from build123d import *

# Parameters (mm, degrees)
SKETCH1_W                = 37
SKETCH1_H                = 37
BOSS_EXTRUDE1_DEPTH      = 2
FILLET1_R                = 3
F_4_0_4_DIAMETER_HOLE1_D = 4
SKETCH6_W                = 28
SKETCH6_H                = 13
BOSS_EXTRUDE3_DEPTH      = 2
SKETCH7_W                = 3
SKETCH7_H                = 13
BOSS_EXTRUDE4_DEPTH      = 3
SKETCH8_W                = 15
SKETCH8_H                = 15
CUT_EXTRUDE1_DEPTH       = 37.653785616


with BuildPart() as part:
    # Sketch1 → Boss-Extrude1 (new body)
    with BuildSketch(Plane(origin=(0, 0, 0), x_dir=(1, 0, 0), z_dir=(0, 1, 0))):
        Rectangle(SKETCH1_W, SKETCH1_H)
    extrude(amount=BOSS_EXTRUDE1_DEPTH)

    # Fillet1
    fillet1_edges = [part.edges().sort_by_distance(p)[0] for p in [
        (-18.5, 1, -18.5),
        (18.5, 1, -18.5),
        (18.5, 1, 18.5),
        (-18.5, 1, 18.5),
    ]]
    fillet(fillet1_edges, radius=FILLET1_R)

    # Ø4.0 (4) Diameter Hole1 (through all)
    with Locations(Plane(origin=(0, 2, 0), x_dir=(1, 0, 0), z_dir=(0, 1, 0))):
        with Locations((-15.25, 15.25), (15.25, -15.25), (15.25, 15.25), (-15.25, -15.25)):
            Hole(F_4_0_4_DIAMETER_HOLE1_D / 2)

    # Sketch6 → Boss-Extrude3 (add, through all)
    with BuildSketch(Plane(origin=(0, 2, 0), x_dir=(1, 0, 0), z_dir=(0, 1, 0))):
        with Locations((0, 25)):
            Rectangle(SKETCH6_W, SKETCH6_H)
    extrude(amount=-BOSS_EXTRUDE3_DEPTH)

    # Sketch7 → Boss-Extrude4 (add)
    with BuildSketch(Plane(origin=(0, 2, 0), x_dir=(1, 0, 0), z_dir=(0, 1, 0))):
        with Locations((-12.5, 25)):
            Rectangle(SKETCH7_W, SKETCH7_H)
        with Locations((12.5, 25)):
            Rectangle(SKETCH7_W, SKETCH7_H)
    extrude(amount=BOSS_EXTRUDE4_DEPTH)

    # Sketch8 → Cut-Extrude1 (cut, through all)
    with BuildSketch(Plane(origin=(0, 2, 0), x_dir=(1, 0, 0), z_dir=(0, 1, 0))):
        with BuildLine():
            Line((7.5, -3.5), (-7.5, -3.5))
            ThreePointArc((-7.5, -3.5), (0, 4), (7.5, -3.5))
        make_face()
        with Locations((0, -11)):
            Rectangle(SKETCH8_W, SKETCH8_H)
    extrude(amount=-CUT_EXTRUDE1_DEPTH, mode=Mode.SUBTRACT)


solid = part.part
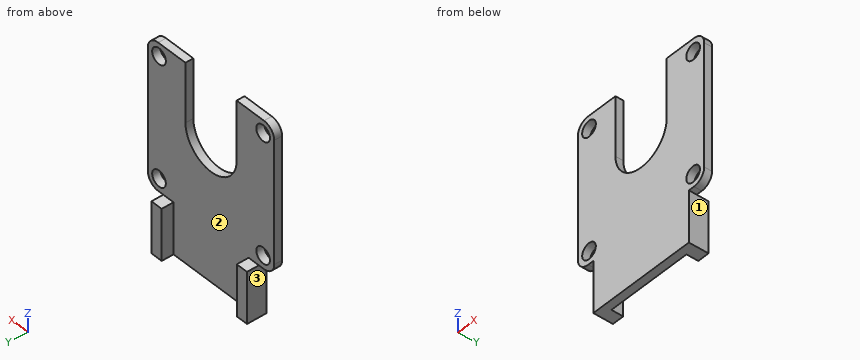
Verification items for the finished model (mm, model axes). Face numbers are marked on the shaded views. Give positions to 0.01 mm unless a question says otherwise; leave off trailing zeros. Order: outer loops, then holes, each group sorted by start corner. A loop starts at its lowest first (then second) coordinate and runs counter-clockwise, first axis right, second up. Notation, with made-up numbers: (76, 23.25) -> (119, 23.25) arc R11 cw to (119, 39.25) -> close; hole circle Ø7 at (83, 82). An arc over 180 degrees is marked (long way). Answer as CSV lines item,"result".
Q1. Sectioned sample at A-A on z = -2.5. Record the cut outline in (x, y), plus the area to 3 significant figures.
Solutions:
outline,"(-18.5, 0) -> (-4.5, 0) -> (-4.5, 2) -> (-18.5, 2) -> close; (4.5, 0) -> (18.5, 0) -> (18.5, 2) -> (4.5, 2) -> close"
area,"56.0 mm²"
Q2. Depth check by flat-ended pin: pin 1 (2.5 mm diameter, centred on y = 2, z = -26, fed in from +X); pin 2 (6 mm diameter, centred on x = 0.5, z = -25, fed in from +Y); pin 3 (0.8 mm diameter, centred on x = 15, y = 1, fed in from -Z); pin 4 (3 mm diameter, centred on x = -15.25, z = 15.25, fed in from +Y) (1 decimal). Enter the tip coordinate at first touch or a pass-through.
Solutions:
pin 1,"stops at x = 14"
pin 2,"stops at y = 2"
pin 3,"stops at z = -18.5"
pin 4,"passes through"
Q3. Sectioned sample at B-B on y = 3.55. Record the cut outline in (x, z), plus the area to 3 significant figures.
Solutions:
outline,"(-14, -31.5) -> (-11, -31.5) -> (-11, -18.5) -> (-14, -18.5) -> close; (11, -31.5) -> (14, -31.5) -> (14, -18.5) -> (11, -18.5) -> close"
area,"78.0 mm²"
Q4. Sectioned sample at D-D on z = -16.5. Record the cut outline in (x, y).
Solutions:
outline,"(-18.33, 0) -> (-16.81, 0) -> (-16.81, 2) -> (-18.33, 2) -> close; (-13.69, 0) -> (13.69, 0) -> (13.69, 2) -> (-13.69, 2) -> close; (16.81, 0) -> (18.33, 0) -> (18.33, 2) -> (16.81, 2) -> close"
Q5. Sectioned sample at C-C on x = 15. Record the cut outline in (y, z), plus the area to 3 significant figures.
Solutions:
outline,"(0, -18.5) -> (2, -18.5) -> (2, -17.23) -> (0, -17.23) -> close; (0, -13.27) -> (2, -13.27) -> (2, 13.27) -> (0, 13.27) -> close; (0, 17.23) -> (2, 17.23) -> (2, 18.5) -> (0, 18.5) -> close"
area,"58.1 mm²"
Q6. Scan lines: probe 1 along Z at (x, y) = (15.25, 1.55); probe 2 along X at (y, z) = (1, 15.25). Record each from-to range of solid material in increasing order.
Solutions:
probe 1,"z = -18.5 to -17.25, -13.25 to 13.25, 17.25 to 18.5"
probe 2,"x = -18.5 to -17.25, -13.25 to -7.5, 7.5 to 13.25, 17.25 to 18.5"
Q7. Release check for a two-part mould opening along X. For the marked faces 1, 2 and 3 record: +X half, -X half, draft (parallel to the pull), parting line (faces both ways), or undercut.
Solutions:
face 1,"+X half"
face 2,"undercut"
face 3,"-X half"
